```python
from build123d import *

# Parameters (mm, degrees)
F0_W     = 11
F0_H     = 23
F1_DEPTH = 6
F2_W     = 9
F2_H     = 4
F3_DEPTH = 23.001
F5_DEPTH = 1.5


with BuildPart() as f1:
    # F0 (on Top) → F1 (new body)
    with BuildSketch(Plane.XY):
        Rectangle(F0_W, F0_H)
    extrude(amount=F1_DEPTH)

    # F2 (on face) → F3 (cut, through all)
    with BuildSketch(Plane.XZ.offset(11.5)):
        with Locations((0, 3)):
            Rectangle(F2_W, F2_H)
    extrude(amount=-F3_DEPTH, mode=Mode.SUBTRACT)

    # F4 (on face) → F5 (cut)
    with BuildSketch(Plane.XY.offset(6)):
        with BuildLine():
            Line((4, 11.5), (-4, 11.5))
            ThreePointArc((-4, 11.5), (0, 7.5), (4, 11.5))
        make_face()
        with BuildLine():
            ThreePointArc((4, -11.5), (0, -7.5), (-4, -11.5))
            Line((-4, -11.5), (4, -11.5))
        make_face()
    extrude(amount=-F5_DEPTH, mode=Mode.SUBTRACT)


solid = f1.part
```
The listing builds one solid part. Answer for the finished solid, in the listing's coordinates (mm). A direction names the side the tool comes from. Coordinates: 2 decimals unless noted, no trailing zeros. Write each loop counter-clockwise with the first axis right and the second up, starting at its lowest first coordinate (ties: lowest second). Pieces come first, ordered by that corner, then holes.
Q1. Section B-B, the plane x = -2.5 is taken. Write down the section's boundary in (y, z), then the cut area to 3 significant figures.
Returned:
outline: (-11.5, 0) - (11.5, 0) - (11.5, 1) - (-11.5, 1) - close; (-8.38, 5) - (8.38, 5) - (8.38, 6) - (-8.38, 6) - close
area: 39.8 mm2
Q2. Section D-D, the plane y = -7.75 is taken. Write down the section's boundary in (x, z).
Returned:
outline: (-5.5, 0) - (5.5, 0) - (5.5, 6) - (1.39, 6) - (1.39, 5) - (4.5, 5) - (4.5, 1) - (-4.5, 1) - (-4.5, 5) - (-1.39, 5) - (-1.39, 6) - (-5.5, 6) - close
Q3. Which of the six approach directions +Z, -Z, +X, -X, +Y, -Y give full straight-line access (tool end or side, diameter ignored) to faces 4 (the flat face through (0, 0, 1)), 5 (the flat face through (-0.1, 11.5, 0.3)), 6 (the cylindrical face through (0.1, -7.5, 5.5))?
Returned:
face 4: +Y, -Y
face 5: +Z, -Z, +X, -X, +Y
face 6: +Z, -Y
Q4. Section C-C, the plane y = 2 is taken. Write down the section's boundary in (x, z), then the cut area to 3 significant figures.
Returned:
outline: (-5.5, 0) - (5.5, 0) - (5.5, 6) - (-5.5, 6) - close; hole (-4.5, 1) - (4.5, 1) - (4.5, 5) - (-4.5, 5) - close
area: 30.0 mm2
Q5. Section A-A, the plane z = 1.6 is taken. Write down the section's boundary in (x, y).
Returned:
outline: (-5.5, -11.5) - (-4.5, -11.5) - (-4.5, 11.5) - (-5.5, 11.5) - close; (4.5, -11.5) - (5.5, -11.5) - (5.5, 11.5) - (4.5, 11.5) - close
Q6. Find the intervals of material crossed by line 1 along Z through (x, y) = (1.5, 4); line 2 along X through (y, z) = (6.75, 1.55), in increasing order.
Returned:
line 1: z = 0 to 1, 5 to 6
line 2: x = -5.5 to -4.5, 4.5 to 5.5
Q7. The mould has two halves that part along X. Classify faces 1 (the cylindrical face through (-0.1, 7.5, 5.5)), 2 (the flat face through (5.5, 0, 3)), 3 (the flat face through (0, 0, 6)): released by +X, released by -X, zero draft, split by the parting line, or undercut.
Returned:
face 1: undercut
face 2: released by +X
face 3: zero draft
